Part model, mm, in its own coordinate system. A direction names the side the tool comes from. Coordinates: 2 decimals unless noted, no trailing zeros. Loops run counter-clockwise (first coordinate to the right, second up) from the corner with the lowest first, then second, coordinate; pieces in that order, holes last. Notation, with made-up numbers: M 80.25,89.25 L 108.25,89.25 A34 ccw 108.25,126.25 Z; hole C 65.5,5.25 d1. An arc over 180 degrees is marked long. Answer as a JSON object with one key per item and string values. Group by question number.
1. Drill centre lines: L1, parallel to X at y = -29, z = -15.5; L2, parallel to X at y = 0, z = -16.75; L3, parallel to Y at x = 0, z = -14.25. Where is each one in solid material? Low to high.
2. 3-axis set-ups, long thin cutter, end or side, ignore diameter. For faces 1 (the face through (-25.19, 15.8, -14.79)), 2 (the face through (2.05, 29.57, -14.79)), 3 (the face through (18.519, 18.548, -15.21)): which of +Z, -Z, +X, -X, +Y, -Y reach the whole face in a straight line?
3. Drop flat-ended pins along their axis: pin 1 Ø1.5 at (x, z) = (-2, -21) entering from -Y; pin 2 Ø3.5 at (y, z) = (19.5, -11) entering from -X; pin 3 Ø1 at (y, z) = (18.5, -9) entering from +X. Give the stop position or say it passes through.
4. Saw through at B-B on x = 0. Write the cut outline in (y, z).
5. Saw through at A-A on y = 0. Write the cut outline in (x, z), then the cut area to 3 significant figures.
6. Mould opens along Y. For faces 4 (the face through (-28.84, 7.24, -14.79)), 5 (the face through (-7.24, -28.84, -14.79)), 6 (the face through (-11.918, 23.344, -15.21)), 7 (the face through (-14, 14, -30)) say: released by +Y, released by -Y, zero draft, split by the parting line, or undercut.
from build123d import *

# Parameters (mm, degrees)
SKETCH1_W           = 8.21
SKETCH1_H           = 30
BOSS_EXTRUDE1_DEPTH = 30
CIRPATTERN1_COUNT   = 20
SKETCH3_W           = 6
SKETCH3_H           = 6
CUT_EXTRUDE1_DEPTH  = 56.479726027


with BuildPart() as part:
    # Sketch1 → Revolve1 (revolve)
    with BuildSketch(Plane(origin=(0, 0, 0), x_dir=(1, 0, 0), z_dir=(0, 1, 0))):
        with Locations((22.105, 15)):
            Rectangle(SKETCH1_W, SKETCH1_H)
    revolve(axis=Axis((0, 0, 0), (0, 0, -1)))

    # Sketch2 → Boss-Extrude1 (add)
    with BuildSketch(Plane.XY):
        with BuildLine():
            ThreePointArc((2.63, 26.077714624), (2.037608033, 29.62132863), (0.79, 32.990542584))
            ThreePointArc((0.79, 32.990542584), (0, 33), (-0.79, 32.990542584))
            ThreePointArc((-0.79, 32.990542584), (-2.037608033, 29.62132863), (-2.63, 26.077714624))
            ThreePointArc((-2.63, 26.077714624), (0, 26.21), (2.63, 26.077714624))
        make_face()
    boss_extrude1 = extrude(amount=-BOSS_EXTRUDE1_DEPTH)

    # CirPattern1: Boss-Extrude1 ×20 about axis
    cirpattern1_axis = Axis((0, 0, 0), (0, 0, 1))
    for i in range(1, CIRPATTERN1_COUNT):
        add(boss_extrude1.rotate(cirpattern1_axis, i * 360 / CIRPATTERN1_COUNT))

    # Sketch3 → Cut-Extrude1 (cut, through all)
    with BuildSketch(Plane.XY):
        with Locations((0, 18)):
            Rectangle(SKETCH3_W, SKETCH3_H)
    extrude(amount=-CUT_EXTRUDE1_DEPTH, mode=Mode.SUBTRACT)


solid = part.part
Outcome:
{
 "1": {"L1": "x = -11.11 to -7.35, -2.19 to 2.19, 7.35 to 11.11", "L2": "x = -33 to -18, 18 to 33", "L3": "y = -33 to -18, 21 to 33"},
 "2": {"face 1": "+Z, -Z, -X", "face 2": "+Z, -Z, +Y", "face 3": "+Z, -Z"},
 "3": {"pin 1": "stops at y = -31.96", "pin 2": "stops at x = -27.15", "pin 3": "stops at x = 27.15"},
 "4": {"outline": "M -33,-30 L -18,-30 L -18,0 L -33,0 Z; M 21,-30 L 33,-30 L 33,0 L 21,0 Z"},
 "5": {"outline": "M -33,-30 L -18,-30 L -18,0 L -33,0 Z; M 18,-30 L 33,-30 L 33,0 L 18,0 Z", "area": "900 mm²"},
 "6": {"face 4": "undercut", "face 5": "released by -Y", "face 6": "undercut", "face 7": "zero draft"}
}
